```python
from build123d import *

# Parameters (mm, degrees)
SZKIC1_W                    = 200
SZKIC1_H                    = 150
DODANIE_WYCI_GNI_CIE1_DEPTH = 10
SZKIC2_W                    = 200
SZKIC2_H                    = 10
DODANIE_WYCI_GNI_CIE2_DEPTH = 50
OTW_R_POD_RUB_M101_D        = 12
SZYK_LINIOWY2_COUNT         = 2
SZYK_LINIOWY2_PITCH         = 150


with BuildPart() as part:
    # Szkic1 → Dodanie-wyciągnięcie1 (new body)
    with BuildSketch(Plane.XY):
        Rectangle(SZKIC1_W, SZKIC1_H)
    extrude(amount=DODANIE_WYCI_GNI_CIE1_DEPTH)

    # Szkic2 → Dodanie-wyciągnięcie2 (add)
    with BuildSketch(Plane.XY.offset(10)):
        with Locations((0, -70)):
            Rectangle(SZKIC2_W, SZKIC2_H)
    extrude(amount=DODANIE_WYCI_GNI_CIE2_DEPTH)

    # Otwór pod śrubę M101 (through all)
    with Locations(Plane(origin=(0, -65, 0), x_dir=(1, 0, 0), z_dir=(0, 1, 0))):
        with Locations((-75, -35)):
            otw_r_pod_rub_m101 = Hole(OTW_R_POD_RUB_M101_D / 2)

    # Szyk liniowy2: Otwór pod śrubę M101 ×2
    with Locations(*[(i * SZYK_LINIOWY2_PITCH, 0, 0) for i in range(1, SZYK_LINIOWY2_COUNT)]):
        add(otw_r_pod_rub_m101, mode=Mode.SUBTRACT)


solid = part.part
```
CAD build for the part. Positions are in the model's coordinates, mm. A direction names the side the tool comes from. Round coordinates to 2 decimals unless told otherwise and drop trailing zeros. Write each loop counter-clockwise with the first axis right and the second up, starting at its lowest first coordinate (ties: lowest second). Pieces come first, ordered by that corner, then holes.
Item 1: Band-saw the part on D-D on y = 15. Write the cut outline in (x, z), then the cut area to 3 significant figures.
Filled in:
outline: (-100, 0) - (100, 0) - (100, 10) - (-100, 10) - close
area: 2,000 mm2
Item 2: Mould opens along Z. For faces 3 (the flat face through (-1, 6, 10)), 4 (the cylindrical face through (-69, -70, 35)), 5 (the cylindrical face through (81, -70, 35)), 6 (the flat face through (-100, -23, 8)) say: released by +Z, released by -Z, zero draft, split by the parting line, or undercut.
Filled in:
face 3: released by +Z
face 4: undercut
face 5: undercut
face 6: zero draft
Item 3: Band-saw the part on B-B on z = 35. Write the cut outline in (x, y).
Filled in:
outline: (-100, -75) - (-81, -75) - (-81, -65) - (-100, -65) - close; (-69, -75) - (69, -75) - (69, -65) - (-69, -65) - close; (81, -75) - (100, -75) - (100, -65) - (81, -65) - close
Item 4: Drop flat-ended pins along their axis: pin 1 Ø10 at (x, z) = (72, 31) entering from +Y; pin 2 Ø1 at (x, y) = (-5.5, -24.5) entering from -Z. Give the stop position or say it passes through.
Filled in:
pin 1: stops at y = -65
pin 2: stops at z = 0
Item 5: Band-saw the part on A-A on x = -75. Write the cut outline in (y, z), then the cut area to 3 significant figures.
Filled in:
outline: (-75, 0) - (75, 0) - (75, 10) - (-65, 10) - (-65, 29) - (-75, 29) - close; (-75, 41) - (-65, 41) - (-65, 60) - (-75, 60) - close
area: 1,880 mm2
Item 6: Tool access for faces 1 (the flat face through (-1, -65, 35)), 2 (the flat face through (-1, 1, 0)): list every direction of +Z, -Z, +X, -X, +Y, -Y with a clear straight run to the whole face (end or side of a thin tool).
Filled in:
face 1: +Z, +X, -X, +Y
face 2: -Z, +X, -X, +Y, -Y
Item 7: Drill centre lines: L1, parallel to X at y = -67.75, z = 35; L2, parallel to Z at x = -75, y = -70.25; L3, parallel to Y at x = -17, z = 55. Where is each one in solid material? Low to high.
Filled in:
L1: x = -100 to -81, -69 to 69, 81 to 100
L2: z = 0 to 29, 41 to 60
L3: y = -75 to -65
Item 8: Band-saw the part on C-C on x = 12. Write the cut outline in (y, z), then the cut area to 3 significant figures.
Filled in:
outline: (-75, 0) - (75, 0) - (75, 10) - (-65, 10) - (-65, 60) - (-75, 60) - close
area: 2,000 mm2
